Model file for the job. Use its own axes, mm. Face numbers are marked on the shaded views. Round coordinates to 2 decimals unless told otherwise and drop trailing zeros. Order: outer loops, then holes, each group sorted by start corner. A loop starts at its lowest first (then second) coordinate and runs counter-clockwise, first axis right, second up. Notation, with made-up numbers: (32.25, -6) - (87.25, -6) arc R13 ccw to (87.25, 6) - close; hole circle Ø11 at (34, 18.25). An arc over 180 degrees is marked (long way). Use one line per item in the form item = value.
from build123d import *

# Parameters (mm, degrees)
BOSS_EXTRUDE1_DEPTH   = 5
F_4_0MM_DOWEL_HOLE1_D = 4


with BuildPart() as part:
    # Sketch1 → Boss-Extrude1 (new body)
    with BuildSketch(Plane.XY):
        with BuildLine():
            Line((5, 17.5), (5, -17.5))
            ThreePointArc((5, -17.5), (0, -22.5), (-5, -17.5))
            Line((-5, -17.5), (-5, 17.5))
            ThreePointArc((-5, 17.5), (0, 22.5), (5, 17.5))
        make_face()
    extrude(amount=BOSS_EXTRUDE1_DEPTH)

    # Ø4.0mm Dowel Hole1 (through all)
    with Locations(Plane.XY.offset(5)):
        with Locations((0, 17.5), (0, -17.5)):
            Hole(F_4_0MM_DOWEL_HOLE1_D / 2)


solid = part.part
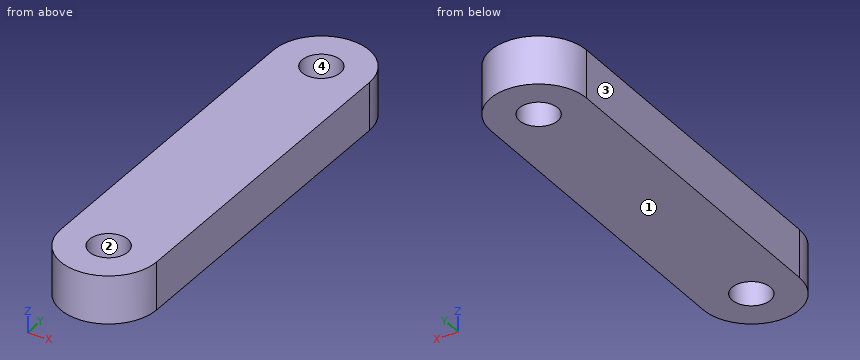
(1) Pin check, flat tips, straight feed: pin 1 (6 mm diameter, centred on x = -1.5, y = 4, fed in from -Z); pin 2 (1.5 mm diameter, centred on x = -3, z = 3, fed in from -Y). Stop position of each tip, or through.
Report:
pin_1 = 0
pin_2 = -21.97
(2) Probe probe 1 along Y at (x, z) = (0, 1.35); probe 2 along Y at (x, z) = (-0.75, 0.5); probe 3 along X at (y, z) = (-16, 3.9). List the from-to ranges inside material, lowest first. Write a range as [from, to].
Report:
probe_1 = [-22.5, -19.5], [-15.5, 15.5], [19.5, 22.5]
probe_2 = [-22.44, -19.35], [-15.65, 15.65], [19.35, 22.44]
probe_3 = [-5, -1.32], [1.32, 5]
(3) Slice it at B-B on x = 0. Give the cut face in (y, z).
Report:
outline = (-22.5, 0) - (-19.5, 0) - (-19.5, 5) - (-22.5, 5) - close; (-15.5, 0) - (15.5, 0) - (15.5, 5) - (-15.5, 5) - close; (19.5, 0) - (22.5, 0) - (22.5, 5) - (19.5, 5) - close
(4) Pull direction X, two halves, no side cores. Call the marked faces 1, 2, 3 and 4: released by +X, released by -X, zero draft, split by the parting line, or undercut.
Report:
face_1 = zero draft
face_2 = undercut
face_3 = released by -X
face_4 = undercut
(5) Slice it at A-A on z = 3.95. Give the cut face in (x, y), then the cut area to 3 significant figures.
Report:
outline = (-5, -17.5) arc R5 ccw to (5, -17.5) - (5, 17.5) arc R5 ccw to (-5, 17.5) - close; hole circle Ø4 at (0, -17.5); hole circle Ø4 at (0, 17.5)
area = 403 mm2
(6) Slice it at C-C on y = 18.5. Give the cut face in (x, z).
Report:
outline = (-4.9, 0) - (-1.73, 0) - (-1.73, 5) - (-4.9, 5) - close; (1.73, 0) - (4.9, 0) - (4.9, 5) - (1.73, 5) - close
(7) Slice it at D-D on x = -4. Give the cut face in (y, z).
Report:
outline = (-20.5, 0) - (20.5, 0) - (20.5, 5) - (-20.5, 5) - close
